Input: part model. Units: mm. Frame: model coordinates. A direction names the side the tool comes from. Coordinates: 2 decimals unless noted, no trailing zeros. Loops run counter-clockwise (first coordinate to the right, second up) from the corner with the lowest first, then second, coordinate; pieces in that order, holes last.
Item 1: Section B-B on z = -1.5. Return loops of the section in (x, y).
Item 2: Reachability of faces 4 (the flat face through (19.941, 1.972, 35.575)), 5 (the cylindrical face through (30.139, 1.972, 21.358)), 6 (the flat face through (-29.788, 1.972, 29.609)), 7 (the flat face through (23.26, 3.01, -23.41)), 8 (the flat face through (35.59, 1.97, 20.03)) from +Z, -Z, +X, -X, +Y, -Y: full face, straight path, thin tool, end or side. Return the list, or none.
Item 3: Section A-A on z = 22.5. Return loops of the section in (x, y), and give its area (3 significant figures).
Item 4: Section D-D on y = 1.1. Give the number of separate pieces and of enclosed holes in the cut face, and give its area (3 significant figures).
Item 5: Ray query, line 1 along Z through (x, y) = (-4, 1.45); line 2 along X through (y, z) = (2.3, 6); line 3 along Z through (x, y) = (18, 2.25). Return the intervals inside material, ascending.
Item 6: Contact query for flat-ended pins moving along their axis: P1, Ø2, axis at y = 1, z = -6.5, coming from the +X side; P2, Ø1, axis at y = 0.5, z = 21, coming from the +X side; P3, Ø2, axis at y = 3, z = -27, coming from the -X side. Output: stop coordinate, or through.
Item 7: Section C-C on x = -26. Return loops of the section in (y, z).
Item 8: Pull-direction query (X, two-part tool) for faces 1 (the flat face through (-33, 4, -1)), 2 (the flat face through (35, 2, 0)), 3 (the cylindrical face through (22.7, 1.97, -32.71)); classes: released by +X, released by -X, zero draft, split by the parting line, or undercut.
```python
from build123d import *

# Parameters (mm, degrees)
SKETCH1_R           = 1.6
BOSS_EXTRUDE1_DEPTH = 4
CUT_EXTRUDE1_DEPTH  = 2
CUT_EXTRUDE2_DEPTH  = 1.5
SKETCH4_R           = 1.5
CUT_EXTRUDE3_DEPTH  = 52.039200621
BOSS_EXTRUDE4_START = 1.5
SKETCH5_R           = 4
SKETCH5_R_2         = 1.5
BOSS_EXTRUDE4_DEPTH = 1.5
CIRPATTERN1_COUNT   = 4
FILLET1_R           = 2
FILLET2_R           = 10


with BuildPart() as part:
    # Sketch1 → Boss-Extrude1 (new body)
    with BuildSketch(Plane(origin=(0, 0, 0), x_dir=(1, 0, 0), z_dir=(0, 1, 0))):
        Polygon((15.934040652, 35), (-15.934040652, 35), (-23.334523779, 36.062445841), (-36.062445841, 23.334523779), (-35, 15.934040652), (-35, -15.934040652), (-36.062445841, -23.334523779), (-23.334523779, -36.062445841), (-15.934040652, -35), (15.934040652, -35), (23.334523779, -36.062445841), (36.062445841, -23.334523779), (35, -15.934040652), (35, 15.934040652), (36.062445841, 23.334523779), (23.334523779, 36.062445841), align=None)
        with Locations(Location((22.627416998, 31.112698372, 0), (0, 0, 270))):
            Circle(SKETCH1_R, mode=Mode.SUBTRACT)
        with Locations(Location((31.112698372, 22.627416998, 0), (0, 0, 270))):
            Circle(SKETCH1_R, mode=Mode.SUBTRACT)
        with Locations(Location((22.627416998, -31.112698372, 0), (0, 0, 270))):
            Circle(SKETCH1_R, mode=Mode.SUBTRACT)
        with Locations(Location((31.112698372, -22.627416998, 0), (0, 0, 270))):
            Circle(SKETCH1_R, mode=Mode.SUBTRACT)
        with Locations(Location((-31.112698372, -22.627416998, 0), (0, 0, 270))):
            Circle(SKETCH1_R, mode=Mode.SUBTRACT)
        with Locations(Location((-22.627416998, -31.112698372, 0), (0, 0, 270))):
            Circle(SKETCH1_R, mode=Mode.SUBTRACT)
        with Locations(Location((-22.627416998, 31.112698372, 0), (0, 0, 270))):
            Circle(SKETCH1_R, mode=Mode.SUBTRACT)
        with Locations(Location((-31.112698372, 22.627416998, 0), (0, 0, 270))):
            Circle(SKETCH1_R, mode=Mode.SUBTRACT)
    extrude(amount=BOSS_EXTRUDE1_DEPTH)

    # Sketch2 → Cut-Extrude1 (cut)
    with BuildSketch(Plane(origin=(0, 4, 0), x_dir=(1, 0, 0), z_dir=(0, 1, 0))):
        Polygon((-17.669047558, 29), (17.669047558, 29), (29, 17.669047558), (29, -17.669047558), (17.669047558, -29), (-17.669047558, -29), (-29, -17.669047558), (-29, 17.669047558), align=None)
    extrude(amount=-CUT_EXTRUDE1_DEPTH, mode=Mode.SUBTRACT)

    # Sketch3 → Cut-Extrude2 (cut)
    with BuildSketch(Plane(origin=(0, 2, 0), x_dir=(1, 0, 0), z_dir=(0, 1, 0))):
        with BuildLine():
            Line((-15, -4.595058717), (-15, 4.595058717))
            ThreePointArc((-15, 4.595058717), (-15.283167889, 5.867388581), (-16.079215521, 6.899529803))
            Line((-16.079215521, 6.899529803), (-24.079215521, 13.567556979))
            ThreePointArc((-24.079215521, 13.567556979), (-27.272329864, 13.979918004), (-29, 11.263085893))
            Line((-29, 11.263085893), (-29, -11.263085893))
            ThreePointArc((-29, -11.263085893), (-27.272329864, -13.979918004), (-24.079215521, -13.567556979))
            Line((-24.079215521, -13.567556979), (-16.079215521, -6.899529803))
            ThreePointArc((-16.079215521, -6.899529803), (-15.283167889, -5.867388581), (-15, -4.595058717))
        make_face()
        with BuildLine():
            Line((-13.567556979, 24.079215521), (-6.899529803, 16.079215521))
            ThreePointArc((-6.899529803, 16.079215521), (-5.867388581, 15.283167889), (-4.595058717, 15))
            Line((-4.595058717, 15), (4.595058717, 15))
            ThreePointArc((4.595058717, 15), (5.867388581, 15.283167889), (6.899529803, 16.079215521))
            Line((6.899529803, 16.079215521), (13.567556979, 24.079215521))
            ThreePointArc((13.567556979, 24.079215521), (13.979918004, 27.272329864), (11.263085893, 29))
            Line((11.263085893, 29), (-11.263085893, 29))
            ThreePointArc((-11.263085893, 29), (-13.979918004, 27.272329864), (-13.567556979, 24.079215521))
        make_face()
        with BuildLine():
            Line((24.079215521, 13.567556979), (16.079215521, 6.899529803))
            ThreePointArc((16.079215521, 6.899529803), (15.283167889, 5.867388581), (15, 4.595058717))
            Line((15, 4.595058717), (15, -4.595058717))
            ThreePointArc((15, -4.595058717), (15.283167889, -5.867388581), (16.079215521, -6.899529803))
            Line((16.079215521, -6.899529803), (24.079215521, -13.567556979))
            ThreePointArc((24.079215521, -13.567556979), (27.272329864, -13.979918004), (29, -11.263085893))
            Line((29, -11.263085893), (29, 11.263085893))
            ThreePointArc((29, 11.263085893), (27.272329864, 13.979918004), (24.079215521, 13.567556979))
        make_face()
        with BuildLine():
            Line((13.567556979, -24.079215521), (6.899529803, -16.079215521))
            ThreePointArc((6.899529803, -16.079215521), (5.867388581, -15.283167889), (4.595058717, -15))
            Line((4.595058717, -15), (-4.595058717, -15))
            ThreePointArc((-4.595058717, -15), (-5.867388581, -15.283167889), (-6.899529803, -16.079215521))
            Line((-6.899529803, -16.079215521), (-13.567556979, -24.079215521))
            ThreePointArc((-13.567556979, -24.079215521), (-13.979918004, -27.272329864), (-11.263085893, -29))
            Line((-11.263085893, -29), (11.263085893, -29))
            ThreePointArc((11.263085893, -29), (13.979918004, -27.272329864), (13.567556979, -24.079215521))
        make_face()
    extrude(amount=-CUT_EXTRUDE2_DEPTH, mode=Mode.SUBTRACT)

    # Sketch4 → Cut-Extrude3 (cut, through all)
    with BuildSketch(Plane(origin=(0, 2, 0), x_dir=(1, 0, 0), z_dir=(0, 1, 0))):
        with Locations(Location((15.25, 15.25, 0), (0, 0, 270))):
            Circle(SKETCH4_R)
    cut_extrude3 = extrude(amount=-CUT_EXTRUDE3_DEPTH, mode=Mode.SUBTRACT)

    # Sketch5 → Boss-Extrude4 (add)
    with BuildSketch(Plane(origin=(0, 2, 0), x_dir=(1, 0, 0), z_dir=(0, 1, 0)).offset(BOSS_EXTRUDE4_START)):
        with Locations(Location((15.25, 15.25, 0), (0, 0, 90))):
            Circle(SKETCH5_R)
        with Locations(Location((15.25, 15.25, 0), (0, 0, 270))):
            Circle(SKETCH5_R_2, mode=Mode.SUBTRACT)
    boss_extrude4 = extrude(amount=-BOSS_EXTRUDE4_DEPTH)

    # CirPattern1: Cut-Extrude3, Boss-Extrude4 ×4 about axis
    cirpattern1_axis = Axis((0, 0, 0), (0, 1, 0))
    add([cut_extrude3.rotate(cirpattern1_axis, i * 360 / CIRPATTERN1_COUNT) for i in range(1, CIRPATTERN1_COUNT)], mode=Mode.SUBTRACT)
    add([boss_extrude4.rotate(cirpattern1_axis, i * 360 / CIRPATTERN1_COUNT) for i in range(1, CIRPATTERN1_COUNT)])

    # Fillet1
    # the kernel refuses this fillet: 2 mm, written as the material it adds along each edge
    with BuildSketch(Plane(origin=(15.25, 2, -15.25), x_dir=(0, 0, -1), z_dir=(1, 0, 0))) as fillet1_piece_1:
        with BuildLine():
            CenterArc((5.936491673, 2), FILLET1_R, 194.477512186, 75.522487814)
            Line((4, 1.5), (3.961270167, 1.49))
            ThreePointArc((3.961270167, 1.49), (3.96, 0.75), (3.96, 0))
            Line((3.96, 0), (4, -0.04))
            Line((4, -0.04), (5.936491673, -0.04))
            Line((5.936491673, -0.04), (5.936491673, 0))
        make_face()
    revolve(axis=Axis((15.25, 2, -15.25), (0, 1, 0)))
    with BuildSketch(Plane(origin=(15.25, 2, 15.25), x_dir=(1, 0, 0), z_dir=(0, 0, 1))) as fillet1_piece_2:
        with BuildLine():
            CenterArc((5.936491673, 2), FILLET1_R, 194.477512186, 75.522487814)
            Line((4, 1.5), (3.961270167, 1.49))
            ThreePointArc((3.961270167, 1.49), (3.96, 0.75), (3.96, 0))
            Line((3.96, 0), (4, -0.04))
            Line((4, -0.04), (5.936491673, -0.04))
            Line((5.936491673, -0.04), (5.936491673, 0))
        make_face()
    revolve(axis=Axis((15.25, 2, 15.25), (0, 1, 0)))
    with BuildSketch(Plane(origin=(-15.25, 2, 15.25), x_dir=(0, 0, 1), z_dir=(-1, 0, 0))) as fillet1_piece_3:
        with BuildLine():
            CenterArc((5.936491673, 2), FILLET1_R, 194.477512186, 75.522487814)
            Line((4, 1.5), (3.961270167, 1.49))
            ThreePointArc((3.961270167, 1.49), (3.96, 0.75), (3.96, 0))
            Line((3.96, 0), (4, -0.04))
            Line((4, -0.04), (5.936491673, -0.04))
            Line((5.936491673, -0.04), (5.936491673, 0))
        make_face()
    revolve(axis=Axis((-15.25, 2, 15.25), (0, 1, 0)))
    with BuildSketch(Plane(origin=(-15.25, 2, -15.25), x_dir=(-1, 0, 0), z_dir=(0, 0, -1))) as fillet1_piece_4:
        with BuildLine():
            CenterArc((5.936491673, 2), FILLET1_R, 194.477512186, 75.522487814)
            Line((4, 1.5), (3.961270167, 1.49))
            ThreePointArc((3.961270167, 1.49), (3.96, 0.75), (3.96, 0))
            Line((3.96, 0), (4, -0.04))
            Line((4, -0.04), (5.936491673, -0.04))
            Line((5.936491673, -0.04), (5.936491673, 0))
        make_face()
    revolve(axis=Axis((-15.25, 2, -15.25), (0, 1, 0)))

    # Fillet2
    fillet2_edges = [part.edges().sort_by_distance(p)[0] for p in [
        (-15.934040652, 2, -35),
        (15.934040652, 2, -35),
        (35, 2, -15.934040652),
        (35, 2, 15.934040652),
        (15.934040652, 2, 35),
        (-15.934040652, 2, 35),
        (-35, 2, 15.934040652),
        (-35, 2, -15.934040652),
    ]]
    fillet(fillet2_edges, radius=FILLET2_R)


solid = part.part
```
Results found:
1. outline: (-35, 0) - (35, 0) - (35, 4) - (29, 4) - (29, 0.5) - (15, 0.5) - (15, 2) - (-15, 2) - (-15, 0.5) - (-29, 0.5) - (-29, 4) - (-35, 4) - close
2. face 4: +Z, +Y, -Y
2. face 5: +Y, -Y
2. face 6: +Z, -X, +Y, -Y
2. face 7: +Y
2. face 8: +X, +Y, -Y
3. outline: (-35.94, 0) - (-32.71, 0) - (-32.71, 4) - (-35.94, 4) - close; (-29.52, 0) - (29.52, 0) - (29.52, 4) - (24.17, 4) - (24.17, 2) - (12.25, 2) - (12.25, 0.5) - (-12.25, 0.5) - (-12.25, 2) - (-24.17, 2) - (-24.17, 4) - (-29.52, 4) - close; (32.71, 0) - (35.94, 0) - (35.94, 4) - (32.71, 4) - close
3. area: 129 mm2
4. separate pieces: 1
4. enclosed holes: 16
4. area: 3,370 mm2
5. line 1: z = -35 to -29, -15 to 15, 29 to 35
5. line 2: x = -35 to -29, 29 to 35
5. line 3: z = -35.3 to -28.67, -19.39 to -11.11, 11.11 to 19.39, 28.67 to 35.3
6. P1: stops at x = 35
6. P2: stops at x = 35.8
6. P3: stops at x = -33.4
7. outline: (0, -33.4) - (4, -33.4) - (4, -20.67) - (2, -20.67) - (2, -14.26) - (0.5, -14.26) - (0.5, 14.26) - (2, 14.26) - (2, 20.67) - (4, 20.67) - (4, 33.4) - (0, 33.4) - close
8. face 1: zero draft
8. face 2: released by +X
8. face 3: undercut
